from build123d import *

# Parameters (mm, degrees)
EXTRUDE_1_DEPTH = 19.5


with BuildPart() as part:
    # 草图1 → 凸台-拉伸1 (new body)
    with BuildSketch(Plane(origin=(0, 0, 0), x_dir=(1, 0, 0), z_dir=(0, 1, 0))):
        with BuildLine():
            Line((-0.536355181, 3.215077001), (-0.536355181, 2.375))
            Line((-0.536355181, 2.375), (-1.575396775, 2.375))
            ThreePointArc((-1.575396775, 2.375), (0, -2.85), (1.575396775, 2.375))
            Line((1.575396775, 2.375), (0.536355181, 2.375))
            Line((0.536355181, 2.375), (0.536355181, 3.215077001))
            Line((0.536355181, 3.215077001), (-0.536355181, 3.215077001))
        make_face()
        with BuildLine():
            ThreePointArc((1.162358254, 1.128416275), (0, -1.62), (-1.162358254, 1.128416275))
            Line((-1.162358254, 1.128416275), (1.162358254, 1.128416275))
        make_face(mode=Mode.SUBTRACT)
    extrude(amount=EXTRUDE_1_DEPTH)


solid = part.part
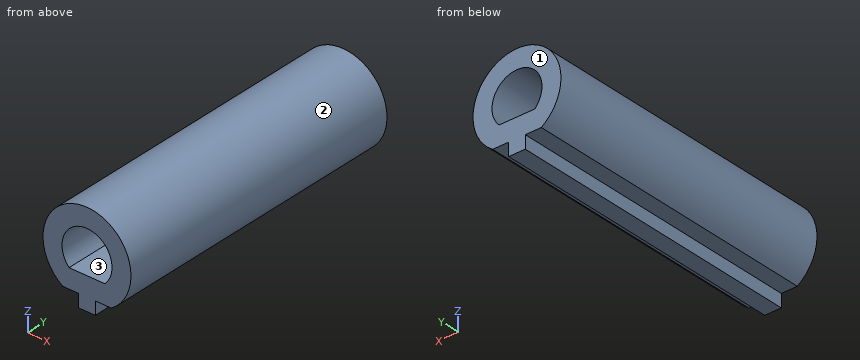
Design review of the part built by this model. Coordinates are the model's own, in mm. Face numbers are marked on the shaded views. Round coordinates to 2 decimals unless told otherwise and drop trailing zeros. Loops run counter-clockwise (first coordinate to the right, second up) from the corner with the lowest first, then second, coordinate; pieces in that order, holes last. Notation, with made-up numbers: M 86.5,2 L 127.5,2 A18 cw 127.5,12 Z; hole C 34.25,49.5 d9. An arc over 180 degrees is marked long. Answer as a JSON object with one key per item and string values.
Item 1: We need section A-A on x = 0. Give the boundary of the cut face in (y, z).
Answer sheet:
{"outline": "M 0,-3.22 L 19.5,-3.22 L 19.5,-1.13 L 0,-1.13 Z; M 0,1.62 L 19.5,1.62 L 19.5,2.85 L 0,2.85 Z"}
Item 2: We need section D-D on z = 2.5. Give the boundary of the cut face in (x, y), and give its area (3 significant figures).
Answer sheet:
{"outline": "M -1.37,0 L 1.37,0 L 1.37,19.5 L -1.37,19.5 Z", "area": "53.4 mm^2"}
Item 3: The part is to be moulded in two halves that separate along Z. For the marked faces 1, 2 and 3, say which applies: pulls with the +Z half, pulls with the -Z half, needs draft (parallel to the pull), parting line crosses it, or undercut.
Answer sheet:
{"face 1": "needs draft", "face 2": "parting line crosses it", "face 3": "undercut"}
Item 4: Wall thickness on L1, parallel to Z at x = 0, y = 12.5; L2, parallel to X at y = 9.5, z = 0; L3, parallel to Z at x = 1.2, y = 14.25 (3 decimals): over which ranges is each line inside the solid? List them lowest first. Write a range as from..to.
Answer sheet:
{"L1": "z = -3.22..-1.13, 1.62..2.85", "L2": "x = -2.85..-1.62, 1.62..2.85", "L3": "z = -2.375..-1.088, 1.088..2.585"}
Item 5: We need section C-C on z = 0. Give the boundary of the cut face in (x, y).
Answer sheet:
{"outline": "M -2.85,0 L -1.62,0 L -1.62,19.5 L -2.85,19.5 Z; M 1.62,0 L 2.85,0 L 2.85,19.5 L 1.62,19.5 Z"}
Item 6: Clearance check with flat-ended pins moving along their axes: P1, Ø0.8, axis at x = -1, y = 7, coming from the -Z side (3 decimals); P2, Ø0.7, axis at y = 14, z = -2.5, coming from the -X side; P3, Ø1, axis at x = -0.5, z = 0.5, coming from the -Y side; P4, Ø0.7, axis at y = 9.5, z = -2.5, coming from the +X side. State where each tip first meets the part, or that it passes through.
Answer sheet:
{"P1": "stops at z = -2.375", "P2": "stops at x = -1.87", "P3": "passes through", "P4": "stops at x = 1.87"}
Item 7: We need section B-B on y = 9.75. Give the boundary of the cut face in (x, z) (3 decimals), and give its area (3 significant figures).
Answer sheet:
{"outline": "M -1.575,-2.375 L -0.536,-2.375 L -0.536,-3.215 L 0.536,-3.215 L 0.536,-2.375 L 1.575,-2.375 A2.85 ccw long Z; hole M -1.162,-1.128 L 1.162,-1.128 A1.62 ccw long Z", "area": "17.9 mm^2"}
